Source: CAD feature listing. Evaluate the final solid. Frame: model axes, mm. Face numbers are marked on the shaded views. A direction names the side the tool comes from. Give positions to 0.01 mm unless a question says otherwise; leave off trailing zeros. Loops run counter-clockwise (first coordinate to the right, second up) from the corner with the lowest first, then second, coordinate; pieces in that order, holes last. Notation, with made-up numbers: (29, 26.25) -> (69, 26.25) arc R18 ccw to (69, 31.25) -> close; hole circle Ø5 at (84, 19). An arc over 180 degrees is marked (long way). Return JSON: item names as keys, results as strings. Group by question number.
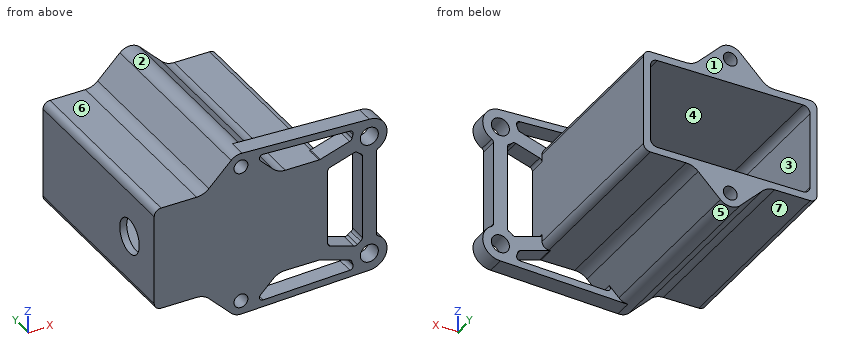
```python
from build123d import *

# Parameters (mm, degrees)
SKETCH1_W           = 50
SKETCH1_H           = 30
BOSS_EXTRUDE1_DEPTH = 3
SKETCH2_W           = 50
SKETCH2_H           = 30
SKETCH2_W_2         = 46
SKETCH2_H_2         = 26
BOSS_EXTRUDE2_DEPTH = 54.15
SKETCH3_R           = 2
BOSS_EXTRUDE3_DEPTH = 57.15
FILLET1_R           = 2
SKETCH4_R           = 5
CUT_EXTRUDE1_DEPTH  = 2
SKETCH5_R           = 2.6
BOSS_EXTRUDE4_DEPTH = 5
FILLET2_R           = 1
FILLET3_R           = 5


with BuildPart() as part:
    # Sketch1 → Boss-Extrude1 (new body)
    with BuildSketch(Plane(origin=(0, 0, 0), x_dir=(1, 0, 0), z_dir=(0, 1, 0))):
        Rectangle(SKETCH1_W, SKETCH1_H)
    extrude(amount=BOSS_EXTRUDE1_DEPTH)

    # Sketch2 → Boss-Extrude2 (add)
    with BuildSketch(Plane(origin=(0, 3, 0), x_dir=(1, 0, 0), z_dir=(0, 1, 0))):
        Rectangle(SKETCH2_W, SKETCH2_H)
        Rectangle(SKETCH2_W_2, SKETCH2_H_2, mode=Mode.SUBTRACT)
    extrude(amount=BOSS_EXTRUDE2_DEPTH)

    # Sketch3 → Boss-Extrude3 (add)
    with BuildSketch(Plane(origin=(0, 0, 0), x_dir=(1, 0, 0), z_dir=(0, 1, 0))):
        with BuildLine():
            ThreePointArc((2.828427125, 22.878427125), (0, 24.05), (-2.828427125, 22.878427125))
            Line((-2.828427125, 22.878427125), (-10.706854249, 15))
            Line((-10.706854249, 15), (10.706854249, 15))
            Line((10.706854249, 15), (2.828427125, 22.878427125))
        make_face()
        with Locations(Location((0, 20.05, 0), (0, 0, 270))):
            Circle(SKETCH3_R, mode=Mode.SUBTRACT)
    boss_extrude3 = extrude(amount=BOSS_EXTRUDE3_DEPTH)

    # Mirror1: Boss-Extrude3 across plane
    add(boss_extrude3.mirror(Plane.XY))

    # Fillet1
    fillet1_edges = [part.edges().sort_by_distance(p)[0] for p in [
        (23, 30.075, 13),
        (23, 30.075, -13),
        (-23, 30.075, -13),
        (-23, 30.075, 13),
        (25, 28.575, 15),
        (-25, 28.575, 15),
        (-25, 28.575, -15),
        (25, 28.575, -15),
    ]]
    fillet(fillet1_edges, radius=FILLET1_R)

    # Sketch4 → Cut-Extrude1 (cut)
    with BuildSketch(Plane.ZY.offset(25)):
        with Locations((0, 12.7)):
            Circle(SKETCH4_R)
    extrude(amount=-CUT_EXTRUDE1_DEPTH, mode=Mode.SUBTRACT)

    # Sketch5 → Boss-Extrude4 (add)
    with BuildSketch(Plane(origin=(0, 0, 0), x_dir=(1, 0, 0), z_dir=(0, 1, 0))):
        with BuildLine():
            Line((3.807606463, 21.899247787), (33.071665812, 20.752413028))
            ThreePointArc((33.071665812, 20.752413028), (32.286385501, 19.447264326), (31.921557121, 17.96842067))
            Line((31.921557121, 17.96842067), (22.686470591, 15))
            Line((22.686470591, 15), (23, 15))
            ThreePointArc((23, 15), (24.414213562, 14.414213562), (25, 13))
            Line((25, 13), (25, 11.542079833))
            Line((25, 11.542079833), (33.145593843, 14.160306425))
            ThreePointArc((33.145593843, 14.160306425), (33.99577787, 13.37875633), (35, 12.808518358))
            Line((35, 12.808518358), (35, -12.808518358))
            ThreePointArc((35, -12.808518358), (33.99577787, -13.37875633), (33.145593843, -14.160306425))
            Line((33.145593843, -14.160306425), (25, -11.542079833))
            Line((25, -11.542079833), (25, -13))
            ThreePointArc((25, -13), (24.414213562, -14.414213562), (23, -15))
            Line((23, -15), (22.686470591, -15))
            Line((22.686470591, -15), (31.921557121, -17.96842067))
            ThreePointArc((31.921557121, -17.96842067), (32.286385501, -19.447264326), (33.071665812, -20.752413028))
            Line((33.071665812, -20.752413028), (3.807606463, -21.899247787))
            Line((3.807606463, -21.899247787), (2.828427125, -22.878427125))
            ThreePointArc((2.828427125, -22.878427125), (1.674272914, -23.682741418), (0.31303276, -24.0377325))
            Line((0.31303276, -24.0377325), (37, -22.6))
            ThreePointArc((37, -22.6), (41.996826812, -18.520647741), (39, -12.808518358))
            Line((39, -12.808518358), (39, 12.808518358))
            ThreePointArc((39, 12.808518358), (41.996826812, 18.520647741), (37, 22.6))
            Line((37, 22.6), (0.31303276, 24.0377325))
            ThreePointArc((0.31303276, 24.0377325), (1.674272914, 23.682741418), (2.828427125, 22.878427125))
            Line((2.828427125, 22.878427125), (3.807606463, 21.899247787))
        make_face()
        with Locations(Location((37, 17.5, 0), (0, 0, 270))):
            Circle(SKETCH5_R, mode=Mode.SUBTRACT)
        with Locations(Location((37, -17.5, 0), (0, 0, 270))):
            Circle(SKETCH5_R, mode=Mode.SUBTRACT)
    extrude(amount=BOSS_EXTRUDE4_DEPTH)

    # Fillet2
    fillet2_edges = [part.edges().sort_by_distance(p)[0] for p in [
        (3.807606463, 2.5, -21.899247787),
        (33.071665812, 2.5, -20.752413028),
        (31.921557121, 2.5, -17.96842067),
        (22.686470591, 2.5, -15),
        (25, 2.5, -11.542079833),
        (33.145593843, 2.5, -14.160306425),
        (35, 2.5, -12.808518358),
        (35, 2.5, 12.808518358),
        (33.145593843, 2.5, 14.160306425),
        (25, 2.5, 11.542079833),
        (22.686470591, 2.5, 15),
        (31.921557121, 2.5, 17.96842067),
        (33.071665812, 2.5, 20.752413028),
        (3.807606463, 2.5, 21.899247787),
        (39, 2.5, 12.808518358),
        (39, 2.5, -12.808518358),
    ]]
    fillet(fillet2_edges, radius=FILLET2_R)

    # Fillet3
    fillet3_edges = [part.edges().sort_by_distance(p)[0] for p in [
        (10.706854249, 28.575, -15),
        (-10.706854249, 28.575, -15),
        (-10.706854249, 28.575, 15),
        (10.706854249, 28.575, 15),
    ]]
    fillet(fillet3_edges, radius=FILLET3_R)


solid = part.part
```
1) Contact query for flat-ended pins moving along their axis: P1, Ø8, axis at x = 10, z = -5, coming from the +Y side; P2, Ø3, axis at x = -15.5, y = 28.5, coming from the -Z side; P3, Ø4, axis at y = 13, z = -16, coming from the -X side; P4, Ø3.5, axis at x = 0, z = -20.05, coming from the +Y side. Output: stop coordinate, or through.
2) Material intervals for line 1 (X direction, y = 14.5, z = 11); line 2 (Y direction, x = -23.7, z = 0); line 3 (Z direction, x = -16, y = 42.5), sorted ascending.
3) Mould query, pull axis X, two halves, no side actions, for the marked faces 1, 2, 3 and 4. Classes: released by +X, released by -X, zero draft, split by the parting line, or undercut.
4) Cut plane A-A on z = 6. Return loops of the section in (x, y).
5) Cut plane B-B on y = 39.5. Count the separate pieces of the cut face and the enclosed holes in it, then the cut area to 3 significant figures.
6) Cut plane C-C on z = -3. Return loops of the section in (x, y), then the cut area to 3 significant figures.
7) Reachability of the marked faces 5, 6 and 7 from +Z, -Z, +X, -X, +Y, -Y: full face, straight path, thin tool, end or side. Return the list, or none.
Calculated:
{
 "1": {"P1": "y = 3", "P2": "z = -15", "P3": "x = -24.73", "P4": "through"},
 "2": {"line 1": "-25 to -23, 23 to 25", "line 2": "0 to 7.7, 17.7 to 57.15", "line 3": "-15 to -13, 13 to 15"},
 "3": {"face 1": "zero draft", "face 2": "split by the parting line", "face 3": "undercut", "face 4": "undercut"},
 "4": {"outline": "(-25, 0) -> (25, 0) -> (25, 57.15) -> (23, 57.15) -> (23, 3) -> (-23, 3) -> (-23, 57.15) -> (-25, 57.15) -> close; (35, 0) -> (39, 0) -> (39, 5) -> (35, 5) -> close"},
 "5": {"separate pieces": "1", "enclosed holes": "3", "area": "503 mm2"},
 "6": {"outline": "(-25, 0) -> (25, 0) -> (25, 57.15) -> (23, 57.15) -> (23, 3) -> (-23, 3) -> (-23, 8.7) -> (-25, 8.7) -> close; (-25, 16.7) -> (-23, 16.7) -> (-23, 57.15) -> (-25, 57.15) -> close; (35, 0) -> (39, 0) -> (39, 5) -> (35, 5) -> close", "area": "371 mm2"},
 "7": {"face 5": "-Z, +Y", "face 6": "+Z, -X, +Y, -Y", "face 7": "-Z, -X, +Y, -Y"}
}
